```python
from build123d import *

# Parameters (mm, degrees)
EXTRUDE_1_DEPTH     = 60
HOLE_WIZARD_2_D     = 24
HOLE_WIZARD_3_D     = 3.2
HOLE_WIZARD_4_D     = 3.2
SKETCH_14_W         = 60
SKETCH_14_H         = 5
CUT_EXTRUDE_1_DEPTH = 5
CHAMFER_1_SIZE      = 2


with BuildPart() as part:
    # 草图1 → 凸台-拉伸1 (new body)
    with BuildSketch(Plane(origin=(0, 0, 0), x_dir=(0, 0, -1), z_dir=(1, 0, 0))):
        Polygon((0, 0), (0, 50), (5, 50), (5, 5), (60, 5), (60, 0), align=None)
    extrude(amount=EXTRUDE_1_DEPTH)

    # 孔2 (through all)
    with Locations(Plane.XY):
        with Locations((30, 26.75)):
            Hole(HOLE_WIZARD_2_D / 2)

    # 孔3 (through all)
    with Locations(Plane.XY):
        with Locations((14.5, 42.25), (45.5, 42.25), (45.5, 11.25), (14.5, 11.25)):
            Hole(HOLE_WIZARD_3_D / 2)

    # 孔4 (through all)
    with Locations(Plane(origin=(0, 5, 0), x_dir=(1, 0, 0), z_dir=(0, 1, 0))):
        with Locations((55.459259259, 14.749042146), (55.459259259, 49.557471264), (4.540740741, 14.749042146), (4.540740741, 49.557471264)):
            Hole(HOLE_WIZARD_4_D / 2)

    # 草图14 → 切除-拉伸1 (cut)
    with BuildSketch(Plane(origin=(0, 0, -60), x_dir=(-1, 0, 0), z_dir=(0, 0, -1))):
        with Locations((-30, 2.5)):
            Rectangle(SKETCH_14_W, SKETCH_14_H)
    extrude(amount=-CUT_EXTRUDE_1_DEPTH, mode=Mode.SUBTRACT)

    # 倒角1
    chamfer_1_edges = [part.edges().sort_by_distance(p)[0] for p in [
        (0, 2.5, -55),
        (60, 50, -2.5),
        (0, 50, -2.5),
        (60, 2.5, -55),
    ]]
    chamfer(chamfer_1_edges, length=CHAMFER_1_SIZE)


solid = part.part
```
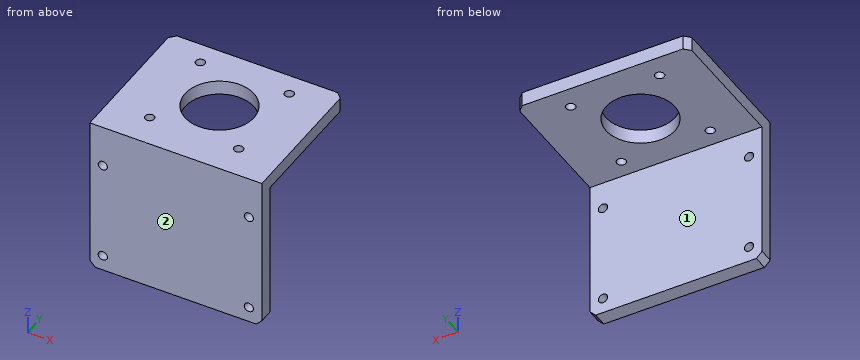
The model under review builds one solid part; all positions refer to its coordinate system, in mm. Face numbers are marked on the shaded views. A direction names the side the tool comes from. Give positions to 0.01 mm unless a question says otherwise; leave off trailing zeros. Write each loop counter-clockwise with the first axis right and the second up, starting at its lowest first coordinate (ties: lowest second). Pieces come first, ordered by that corner, then holes. Notation, with made-up numbers: M 89.25,77.5 L 114.25,77.5 A10 ccw 114.25,81.5 Z; hole C 80,37.5 d1. An arc over 180 degrees is marked long. Write item = value, one per line. Start each with the question number.
Q1. We need section C-C (x = 45.5). State the section outline as (y, z) points, plus the area to 3 significant figures.
Q2. For line 1 (Y direction, x = 45.5, z = -2.1); line 2 (X direction, y = 11, z = -2); line 3 (Y direction, x = 30, z = -1), list the stretches that pass through material, from the lowest coordinate up.
Q3. Clearance check with flat-ended pins moving along their axes: pin 1 (8 mm diameter, centred on x = 18, z = -35.5, fed in from +Y); pin 2 (3 mm diameter, centred on x = 55.46, z = -49.56, fed in from +Y); pin 3 (1.5 mm diameter, centred on x = 8.5, y = 43.5, fed in from -Z). State where each tip first meets the part, or that it passes through.
Q4. We need section B-B (y = 26.75). State the section outline as (x, z) points, plus the area to 3 significant figures.
Q5. We need section D-D (y = 42.25). State the section outline as (x, z) points, plus the area to 3 significant figures.
Q6. We need section A-A (x = 30). State the section outline as (y, z) points.
Q7. Machinability: for the marked faces 1 and 2, which of the approach directions +Z, -Z, +X, -X, +Y, -Y give a long, thin tool a straight path to every point of the face, cutting with its end or side? Answer none if there is none.
Result set:
q1.outline = M 0,-55 L 5,-55 L 5,-5 L 9.65,-5 L 9.65,0 L 0,0 Z; M 12.85,-5 L 40.65,-5 L 40.65,0 L 12.85,0 Z; M 43.85,-5 L 50,-5 L 50,0 L 43.85,0 Z
q1.area = 468 mm2
q2.line_1 = 0 to 9.65, 12.85 to 40.65, 43.85 to 50
q2.line_2 = 0 to 12.92, 16.08 to 43.92, 47.08 to 60
q2.line_3 = 0 to 14.75, 38.75 to 50
q3.pin_1 = 5
q3.pin_2 = through
q3.pin_3 = -5
q4.outline = M 0,-5 L 18,-5 L 18,0 L 0,0 Z; M 42,-5 L 60,-5 L 60,0 L 42,0 Z
q4.area = 180 mm2
q5.outline = M 0,-5 L 12.9,-5 L 12.9,0 L 0,0 Z; M 16.1,-5 L 43.9,-5 L 43.9,0 L 16.1,0 Z; M 47.1,-5 L 60,-5 L 60,0 L 47.1,0 Z
q5.area = 268 mm2
q6.outline = M 0,-55 L 5,-55 L 5,-5 L 14.75,-5 L 14.75,0 L 0,0 Z; M 38.75,-5 L 50,-5 L 50,0 L 38.75,0 Z
q7.face_1 = -Z, +X, -X, +Y
q7.face_2 = +Z, -Z, +X, -X, -Y
